Part model, mm, in its own coordinate system. Face numbers are marked on the shaded views. Give positions to 0.01 mm unless a question says otherwise; leave off trailing zeros. Write each loop counter-clockwise with the first axis right and the second up, starting at its lowest first coordinate (ties: lowest second). Pieces come first, ordered by that corner, then holes.
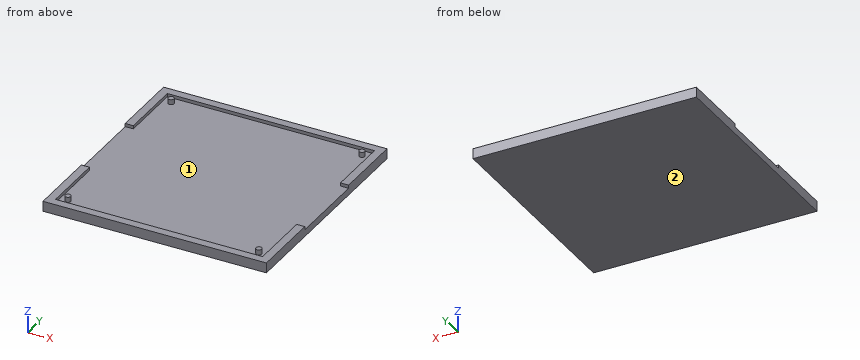
from build123d import *

# Parameters (mm, degrees)
SKETCH1_W           = 110
SKETCH1_H           = 110
BOSS_EXTRUDE1_DEPTH = 5
SKETCH3_W           = 102
SKETCH3_H           = 102
CUT_EXTRUDE1_DEPTH  = 1.6
SKETCH4_R           = 1.4
BOSS_EXTRUDE3_DEPTH = 2.5
SKETCH11_W          = 5
SKETCH11_H          = 40
CUT_EXTRUDE3_DEPTH  = 1.6


with BuildPart() as part:
    # Sketch1 → Boss-Extrude1 (new body)
    with BuildSketch(Plane(origin=(0, 0, 0), x_dir=(1, 0, 0), z_dir=(0, 0, -1))):
        with Locations((55, 55)):
            Rectangle(SKETCH1_W, SKETCH1_H)
    extrude(amount=-BOSS_EXTRUDE1_DEPTH)

    # Sketch3 → Cut-Extrude1 (cut)
    with BuildSketch(Plane(origin=(0, 0, 5), x_dir=(-1, 0, 0), z_dir=(0, 0, 1))):
        with Locations((-55, 55)):
            Rectangle(SKETCH3_W, SKETCH3_H)
    extrude(amount=-CUT_EXTRUDE1_DEPTH, mode=Mode.SUBTRACT)

    # Sketch4 → Boss-Extrude3 (add)
    with BuildSketch(Plane(origin=(0, 0, 3.4), x_dir=(-1, 0, 0), z_dir=(0, 0, 1))):
        with Locations((-102, 102)):
            Circle(SKETCH4_R)
        with Locations((-8, 102)):
            Circle(SKETCH4_R)
        with Locations((-102, 8)):
            Circle(SKETCH4_R)
        with Locations((-8, 8)):
            Circle(SKETCH4_R)
    extrude(amount=BOSS_EXTRUDE3_DEPTH)

    # Sketch11 → Cut-Extrude3 (cut)
    with BuildSketch(Plane(origin=(0, 0, 5), x_dir=(-1, 0, 0), z_dir=(0, 0, 1))):
        with Locations((-108.5, 55)):
            Rectangle(SKETCH11_W, SKETCH11_H)
        with Locations((-1.5, 55)):
            Rectangle(SKETCH11_W, SKETCH11_H)
    extrude(amount=-CUT_EXTRUDE3_DEPTH, mode=Mode.SUBTRACT)


solid = part.part
1) Saw through at C-C (x = 8). Write the cut outline in (y, z).
Check result:
outline: (-110, 0) - (0, 0) - (0, 5) - (-4, 5) - (-4, 3.4) - (-6.6, 3.4) - (-6.6, 5.9) - (-9.4, 5.9) - (-9.4, 3.4) - (-100.6, 3.4) - (-100.6, 5.9) - (-103.4, 5.9) - (-103.4, 3.4) - (-106, 3.4) - (-106, 5) - (-110, 5) - close
2) Drill centre lines: L1, parallel to X at y = -12, z = 4.1; L2, parallel to Y at x = 21.5, z = 3.75; L3, parallel to Z at x = 14, y = -78. Where is each one in solid material? Low to high.
Check result:
L1: x = 0 to 4, 106 to 110
L2: y = -110 to -106, -4 to 0
L3: z = 0 to 3.4
3) Saw through at B-B (x = 53). Write the cut outline in (y, z).
Check result:
outline: (-110, 0) - (0, 0) - (0, 5) - (-4, 5) - (-4, 3.4) - (-106, 3.4) - (-106, 5) - (-110, 5) - close
4) Saw through at D-D (y = -102). Write the cut outline in (x, z).
Check result:
outline: (0, 0) - (110, 0) - (110, 5) - (106, 5) - (106, 3.4) - (103.4, 3.4) - (103.4, 5.9) - (100.6, 5.9) - (100.6, 3.4) - (9.4, 3.4) - (9.4, 5.9) - (6.6, 5.9) - (6.6, 3.4) - (4, 3.4) - (4, 5) - (0, 5) - close
5) Saw through at A-A (y = -85). Write the cut outline in (x, z).
Check result:
outline: (0, 0) - (110, 0) - (110, 5) - (106, 5) - (106, 3.4) - (4, 3.4) - (4, 5) - (0, 5) - close
6) Mould opens along X. For the marked faces 1 and 2 say: +X half, -X half, draft (parallel to the pull), parting line (faces both ways), or undercut.
Check result:
face 1: undercut
face 2: draft
